from build123d import *

# Parameters (mm, degrees)
SKETCH1_W                        = 100
SKETCH1_H                        = 100
BOSS_EXTRUDE1_DEPTH              = 5
F_25_0_25_DIAMETER_HOLE1_D       = 25
F_25_0_25_DIAMETER_HOLE1_DEPTH   = 5
CBORE_FOR_M1_6_SHCS1_D           = 1.7
CBORE_FOR_M1_6_SHCS1_DEPTH       = 5
CBORE_FOR_M1_6_SHCS1_CBORE_D     = 3.5
CBORE_FOR_M1_6_SHCS1_CBORE_DEPTH = 1.6
M1_6X0_35_TAPPED_HOLE1_D         = 1.25
M1_6X0_35_TAPPED_HOLE1_DEPTH     = 5
CBORE_FOR_M3_SHCS1_D             = 3.2
CBORE_FOR_M3_SHCS1_DEPTH         = 5
CBORE_FOR_M3_SHCS1_CBORE_D       = 6.5
CBORE_FOR_M3_SHCS1_CBORE_DEPTH   = 3
F_3_0MM_DOWEL_HOLE1_D            = 3
F_3_0MM_DOWEL_HOLE1_DEPTH        = 4.5
F_3_0MM_DOWEL_HOLE1_TIP          = 0.901290929
CBORE_FOR_M4_SHCS3_D             = 4.3
CBORE_FOR_M4_SHCS3_DEPTH         = 5
CBORE_FOR_M4_SHCS3_CBORE_D       = 8
CBORE_FOR_M4_SHCS3_CBORE_DEPTH   = 4
F_4_0MM_DOWEL_HOLE1_D            = 4
F_4_0MM_DOWEL_HOLE1_DEPTH        = 4
M2X0_4_TAPPED_HOLE1_D            = 1.6
M2X0_4_TAPPED_HOLE1_DEPTH        = 5.2
M2X0_4_TAPPED_HOLE1_TIP          = 0.480688495
M2X0_4_TAPPED_HOLE2_D            = 1.6
M2X0_4_TAPPED_HOLE2_DEPTH        = 5.2
M2X0_4_TAPPED_HOLE2_TIP          = 0.480688495


with BuildPart() as part:
    # Sketch1 → Boss-Extrude1 (new body)
    with BuildSketch(Plane(origin=(0, 0, 0), x_dir=(1, 0, 0), z_dir=(0, 1, 0))):
        Rectangle(SKETCH1_W, SKETCH1_H)
    extrude(amount=BOSS_EXTRUDE1_DEPTH)

    # Ø25.0 (25) Diameter Hole1
    with Locations(Plane(origin=(0, 5, 0), x_dir=(1, 0, 0), z_dir=(0, 1, 0))):
        with Locations((-21.874935549, 17.227744249)):
            Hole(F_25_0_25_DIAMETER_HOLE1_D / 2, depth=F_25_0_25_DIAMETER_HOLE1_DEPTH)

    # CBORE for M1.6 SHCS1
    with Locations(Plane(origin=(0, 5, 0), x_dir=(1, 0, 0), z_dir=(0, 1, 0))):
        with Locations((-32, 35.504948403), (-22, 35.504948403), (-12, 35.504948403), (-2, 35.504948403), (8, 35.504948403), (18, 35.504948403), (18, -3.495051597), (8, -3.495051597), (-2, -3.495051597), (-12, -3.495051597), (-22, -3.495051597), (-32, -3.495051597)):
            CounterBoreHole(CBORE_FOR_M1_6_SHCS1_D / 2, CBORE_FOR_M1_6_SHCS1_CBORE_D / 2, CBORE_FOR_M1_6_SHCS1_CBORE_DEPTH, depth=CBORE_FOR_M1_6_SHCS1_DEPTH)

    # M1.6x0.35 Tapped Hole1
    with Locations(Plane(origin=(0, 0, 0), x_dir=(-1, 0, 0), z_dir=(0, -1, 0))):
        with Locations((37.961945314, 5.5), (-22.961945314, 5.5)):
            Hole(M1_6X0_35_TAPPED_HOLE1_D / 2, depth=M1_6X0_35_TAPPED_HOLE1_DEPTH)

    # CBORE for M3 SHCS1
    with Locations(Plane(origin=(0, 5, 0), x_dir=(1, 0, 0), z_dir=(0, 1, 0))):
        with Locations((-19.518211542, 46.528144303), (-45.766139787, 16.455389216), (-17.50826472, -12.046305538)):
            CounterBoreHole(CBORE_FOR_M3_SHCS1_D / 2, CBORE_FOR_M3_SHCS1_CBORE_D / 2, CBORE_FOR_M3_SHCS1_CBORE_DEPTH, depth=CBORE_FOR_M3_SHCS1_DEPTH)

    # Ø3.0mm Dowel Hole1
    with Locations(Plane(origin=(0, 0, 0), x_dir=(-1, 0, 0), z_dir=(0, -1, 0))):
        with Locations((3.5, -12.04), (34.5, -12.04), (45.75, -3.54), (45.75, 38), (34.5, 46.5), (3.5, 46.5)):
            Hole(F_3_0MM_DOWEL_HOLE1_D / 2, depth=F_3_0MM_DOWEL_HOLE1_DEPTH)
            with Locations((0, 0, -(F_3_0MM_DOWEL_HOLE1_DEPTH + F_3_0MM_DOWEL_HOLE1_TIP / 2))):  # 118° drill point
                Cone(0, F_3_0MM_DOWEL_HOLE1_D / 2, F_3_0MM_DOWEL_HOLE1_TIP, mode=Mode.SUBTRACT)

    # CBORE for M4 SHCS3
    with Locations(Plane(origin=(0, 0, 0), x_dir=(-1, 0, 0), z_dir=(0, -1, 0))):
        with Locations((28.876959135, -33.77675291), (-28.120192829, -15.777088357)):
            CounterBoreHole(CBORE_FOR_M4_SHCS3_D / 2, CBORE_FOR_M4_SHCS3_CBORE_D / 2, CBORE_FOR_M4_SHCS3_CBORE_DEPTH, depth=CBORE_FOR_M4_SHCS3_DEPTH)

    # Ø4.0mm Dowel Hole1
    with Locations(Plane(origin=(0, 5, 0), x_dir=(1, 0, 0), z_dir=(0, 1, 0))):
        with Locations((-28.874935549, -15.772255751), (28.125064451, -33.772255751)):
            Hole(F_4_0MM_DOWEL_HOLE1_D / 2, depth=F_4_0MM_DOWEL_HOLE1_DEPTH)

    # M2x0.4 Tapped Hole1
    with Locations(Plane(origin=(0, 0, -50), x_dir=(-1, 0, 0), z_dir=(0, 0, -1))):
        with Locations((-27.556293219, 2.5)):
            Hole(M2X0_4_TAPPED_HOLE1_D / 2, depth=M2X0_4_TAPPED_HOLE1_DEPTH)
            with Locations((0, 0, -(M2X0_4_TAPPED_HOLE1_DEPTH + M2X0_4_TAPPED_HOLE1_TIP / 2))):  # 118° drill point
                Cone(0, M2X0_4_TAPPED_HOLE1_D / 2, M2X0_4_TAPPED_HOLE1_TIP, mode=Mode.SUBTRACT)

    # M2x0.4 Tapped Hole2
    with Locations(Plane(origin=(50, 0, 0), x_dir=(0, 0, -1), z_dir=(1, 0, 0))):
        with Locations((-4.832893219, 2.5), (39.292893219, 2.5)):
            Hole(M2X0_4_TAPPED_HOLE2_D / 2, depth=M2X0_4_TAPPED_HOLE2_DEPTH)
            with Locations((0, 0, -(M2X0_4_TAPPED_HOLE2_DEPTH + M2X0_4_TAPPED_HOLE2_TIP / 2))):  # 118° drill point
                Cone(0, M2X0_4_TAPPED_HOLE2_D / 2, M2X0_4_TAPPED_HOLE2_TIP, mode=Mode.SUBTRACT)


solid = part.part
For this review, take the finished solid that the model builds, in its own axes (mm). A direction names the side the tool comes from. Round coordinates to 2 decimals unless told otherwise and drop trailing zeros. Write each loop counter-clockwise with the first axis right and the second up, starting at its lowest first coordinate (ties: lowest second). Pieces come first, ordered by that corner, then holes. Notation, with made-up numbers: (49.5, -0.75) - (92.5, -0.75) arc R33 cw to (92.5, 36.25) - close; hole circle Ø10 at (-40, 75.5). An arc over 180 degrees is marked (long way). Write item = value, one per line. Start each with the question number.
1. Draft analysis for pull direction X (two halves, no side actions). For faces 1 (the face through (-11, 3.4, 3)), 2 (the face through (-29.343, 4.507, 35.876)), state which applies: released by +X, released by -X, zero draft, split by the parting line, or undercut.
2. Consider section A-A on z = -8. State the section outline as (x, y) points.
3. For pin 1 Ø1.8 at (x, z) = (18.5, 3) entering from +Y; pin 2 Ø2 at (x, z) = (-29.5, 15.5) entering from +Y, all flat-tipped, find the tip position at first contact; note any pin that passes through.
4. For faces 3 (the face through (-3.825, 2.281, -45.036)), 4 (the face through (-2.4, 4.2, -33.8)), 5 (the face through (-20.25, 2.46, -29.62)), list the 3-axis set-ups (+Z, -Z, +X, -X, +Y, -Y) from which the entire face can be reached by the end or side of a thin tool; tool diameter is ignored.
5. Wall thickness on L1, parallel to Z at x = -45.75, y = 2.1; L2, parallel to X at y = 1.9, z = 33.5; L3, parallel to Z at x = -12, y = 4.5: over which ranges is each line inside the solid? List them lowest first.
Evaluation:
q1.face_1 = undercut
q1.face_2 = undercut
q2.outline = (-50, 0) - (-30.31, 0) - (-30.31, 5) - (-50, 5) - close; (-13.44, 0) - (50, 0) - (50, 5) - (-13.44, 5) - close
q3.pin_1 = 3.4
q3.pin_2 = 1
q4.face_3 = -Y
q4.face_4 = +Y
q4.face_5 = +Y, -Y
q5.L1 = -50 to -39.5, -36.5 to -19.71, -13.21 to 2.04, 5.04 to 50
q5.L2 = -50 to -32.87, -24.89 to 26.14, 30.11 to 50
q5.L3 = -50 to -37.25, -33.75 to -24.89, -9.56 to 1.75, 5.25 to 50
